Geometry check sheet. Reference: the model listing, model coordinates, mm. Round coordinates to 2 decimals unless told otherwise and drop trailing zeros. Write each loop counter-clockwise with the first axis right and the second up, starting at its lowest first coordinate (ties: lowest second). Pieces come first, ordered by that corner, then holes. Notation, with made-up numbers: (-14.5, 5.5) -> (24.5, 5.5) arc R28 ccw to (24.5, 41.5) -> close; hole circle Ø7 at (-35, 78). An arc over 180 degrees is marked (long way). Return JSON: item names as keys, results as strings. Group by question number.
from build123d import *

# Parameters (mm, degrees)
SKETCH_1_R      = 42.5
SKETCH_1_R_2    = 2
EXTRUDE_1_DEPTH = 5


with BuildPart() as part:
    # ｽｹｯﾁ1 → ﾎﾞｽ - 押し出し1 (new body)
    with BuildSketch(Plane(origin=(0, 0, 0), x_dir=(1, 0, 0), z_dir=(0, 1, 0))):
        with Locations(Location((0, 0, 0), (0, 0, 270))):
            Circle(SKETCH_1_R)
        with Locations(Location((5.303300859, 5.303300859, 0), (0, 0, 270))):
            Circle(SKETCH_1_R_2, mode=Mode.SUBTRACT)
        with Locations(Location((5.303300859, -5.303300859, 0), (0, 0, 270))):
            Circle(SKETCH_1_R_2, mode=Mode.SUBTRACT)
        with Locations(Location((-5.303300859, -5.303300859, 0), (0, 0, 270))):
            Circle(SKETCH_1_R_2, mode=Mode.SUBTRACT)
        with Locations(Location((-5.303300859, 5.303300859, 0), (0, 0, 270))):
            Circle(SKETCH_1_R_2, mode=Mode.SUBTRACT)
        with Locations(Location((25, 0, 0), (0, 0, 270))):
            Circle(SKETCH_1_R_2, mode=Mode.SUBTRACT)
        with Locations(Location((0, -25, 0), (0, 0, 270))):
            Circle(SKETCH_1_R_2, mode=Mode.SUBTRACT)
        with Locations(Location((-25, 0, 0), (0, 0, 270))):
            Circle(SKETCH_1_R_2, mode=Mode.SUBTRACT)
        with Locations(Location((0, 25, 0), (0, 0, 270))):
            Circle(SKETCH_1_R_2, mode=Mode.SUBTRACT)
        with Locations(Location((35, 12.5, 0), (0, 0, 270))):
            Circle(SKETCH_1_R_2, mode=Mode.SUBTRACT)
        with Locations(Location((35, -12.5, 0), (0, 0, 270))):
            Circle(SKETCH_1_R_2, mode=Mode.SUBTRACT)
        with Locations(Location((-35, -12.5, 0), (0, 0, 270))):
            Circle(SKETCH_1_R_2, mode=Mode.SUBTRACT)
        with Locations(Location((-35, 12.5, 0), (0, 0, 270))):
            Circle(SKETCH_1_R_2, mode=Mode.SUBTRACT)
    extrude(amount=EXTRUDE_1_DEPTH)


solid = part.part
1) Sectioned sample at D-D on x = 24. Enter the section's corners in (y, z), and give its area (3 significant figures).
2) Go/stop test with flat-tipped pins: P1, Ø2, axis at x = -2, y = 2.5, coming from the -Z side; P2, Ø2, axis at x = -7, y = 3, coming from the -Z side; P3, Ø2, axis at y = 2, z = -10, coming from the -X side. Record where each tip stops, or that it passes through.
3) Sectioned sample at B-B on x = 35. Enter the section's corners in (y, z).
4) Sectioned sample at A-A on z = 26. Enter the section's corners in (x, y).
5) Mould release check, pull along Z, two halves, no side actions. Record for faces 1 (the face through (-25.861, 2.465, -33.727)), 2 (the face through (1, 0, -1)), 3 (the face through (-36.952, 2.465, -12.934)): +Z half, -Z half, draft (parallel to the pull), parting line (faces both ways), or undercut.
6) Sectioned sample at C-C on y = 1.55. State how many separate pieces and enclosed holes the cut face has, and give its area (3 significant figures).
7) Material ranges on probe 1 along X at (y, z) = (0.75, 3.5); probe 2 along Z at (x, y) = (-0.5, 2.8), recorded low to high. Write a range as [from, to].
Evaluation:
{
 "1": {"outline": "(0, -35.07) -> (5, -35.07) -> (5, -1.73) -> (0, -1.73) -> close; (0, 1.73) -> (5, 1.73) -> (5, 35.07) -> (0, 35.07) -> close", "area": "333 mm2"},
 "2": {"P1": "stops at z = -42.49", "P2": "stops at z = -42.07", "P3": "stops at x = -41.54"},
 "3": {"outline": "(0, -24.11) -> (5, -24.11) -> (5, -14.5) -> (0, -14.5) -> close; (0, -10.5) -> (5, -10.5) -> (5, 10.5) -> (0, 10.5) -> close; (0, 14.5) -> (5, 14.5) -> (5, 24.11) -> (0, 24.11) -> close"},
 "4": {"outline": "(-33.62, 0) -> (-1.73, 0) -> (-1.73, 5) -> (-33.62, 5) -> close; (1.73, 0) -> (33.62, 0) -> (33.62, 5) -> (1.73, 5) -> close"},
 "5": {"face 1": "parting line", "face 2": "draft", "face 3": "undercut"},
 "6": {"separate pieces": "1", "enclosed holes": "12", "area": "5,520 mm2"},
 "7": {"probe 1": "x = [-42.36, -6.17], [-4.44, 4.44], [6.17, 42.36]", "probe 2": "z = [-42.5, -26.94], [-23.06, 23.06], [26.94, 42.5]"}
}
